Here's how the part is built. I have some questions about the finished solid (model axes, mm). A direction names the side the tool comes from. Give positions to 0.01 mm unless a question says otherwise; leave off trailing zeros. Order: outer loops, then holes, each group sorted by start corner. A loop starts at its lowest first (then second) coordinate and runs counter-clockwise, first axis right, second up.
from build123d import *

# Parameters (mm, degrees)
F0_W     = 180
F0_H     = 150
F1_DEPTH = 20
F2_R     = 4
F3_DEPTH = 10
F4_W     = 20
F4_H     = 150
F5_DEPTH = 10
F6_ANGLE = 90


with BuildPart() as f1:
    # F0 (on Front) → F1 (new body)
    with BuildSketch(Plane.XZ):
        with Locations((-90, 75)):
            Rectangle(F0_W, F0_H)
    extrude(amount=F1_DEPTH)

    # F2 (on face) → F3 (cut)
    with BuildSketch(Plane.XZ.offset(20)):
        with Locations((-10, 105)):
            Circle(F2_R)
        with Locations((-10, 75)):
            Circle(F2_R)
        with Locations((-10, 45)):
            Circle(F2_R)
    extrude(amount=-F3_DEPTH, mode=Mode.SUBTRACT)

    # F4 (on face) → F5 (cut)
    with BuildSketch(Plane.XZ.offset(20)):
        with Locations((-170, 75)):
            Rectangle(F4_W, F4_H)
    extrude(amount=-F5_DEPTH, mode=Mode.SUBTRACT)


with BuildPart() as f1_1:
    # F6: moved
    add(f1.part.rotate(Axis((-180, 0, 75), (0, 0, 1)), F6_ANGLE))


solid = f1_1.part
Q1. If we section it at A-A on x = -166: List the corners of the cut face in (y, z) for me.
Filled sheet:
outline: (20, 0) - (180, 0) - (180, 150) - (20, 150) - close; hole circle Ø8 at (170, 45); hole circle Ø8 at (170, 75); hole circle Ø8 at (170, 105)
Q2. Thinking about a two-plate mould opening in Y: for faces 4 (the face through (-164.93, 173.815, 46.201)), 5 (the face through (-170, 180, 74)), 6 (the face through (-165, 20, 74)), 7 (the face through (-160, 99, 76)), which applies, released by +Y, released by -Y, zero draft, split by the parting line, or undercut?
Filled sheet:
face 4: undercut
face 5: released by +Y
face 6: released by -Y
face 7: zero draft
Q3. If we section it at D-D on y = 13: List the corners of the cut face in (x, z) for me, plus the area to 3 significant figures.
Filled sheet:
outline: (-180, 0) - (-170, 0) - (-170, 150) - (-180, 150) - close
area: 1,500 mm2
Q4. If we section it at B-B on z = 75: List the corners of the cut face in (x, y) for me.
Filled sheet:
outline: (-180, 0) - (-170, 0) - (-170, 20) - (-160, 20) - (-160, 166) - (-170, 166) - (-170, 174) - (-160, 174) - (-160, 180) - (-180, 180) - close
Q5. For faces 1 (the face through (-170, 10, 76)), 2 (the face through (-170, 89, 0)), 3 (the face through (-170, 170, 45)), which set-ups out of +Z, -Z, +X, -X, +Y, -Y let a thin tool reach every point of the face, with its end or its side?
Filled sheet:
face 1: +Z, -Z, +X, -Y
face 2: -Z, +X, -X, +Y, -Y
face 3: +X
Q6. I need wall thicknesses on L1, parallel to Z at x = -167, y = 170; L2, parallel to Y at x = -165.25, z = 104.5; L3, parallel to Z at x = -169.5, y = 171.5. Which ranges of each line are inside material? Lowest first, please.
Filled sheet:
L1: z = 0 to 41, 49 to 71, 79 to 101, 109 to 150
L2: y = 20 to 166.03, 173.97 to 180
L3: z = 0 to 41.29, 48.71 to 71.29, 78.71 to 101.29, 108.71 to 150
Q7. I'm going to push flat-ended pins straight in: P1, Ø22, axis at y = 5.5, z = 66.5, coming from the +X side; P2, Ø3, axis at x = -165.5, z = 78.5, coming from the -Y side. Where does each tip first touch, or does it pass through?
Filled sheet:
P1: stops at x = -170
P2: stops at y = 20
Q8. If we section it at C-C on y = 170: List the corners of the cut face in (x, z) for me, plus the area to 3 significant figures.
Filled sheet:
outline: (-180, 0) - (-160, 0) - (-160, 41) - (-170, 41) - (-170, 49) - (-160, 49) - (-160, 71) - (-170, 71) - (-170, 79) - (-160, 79) - (-160, 101) - (-170, 101) - (-170, 109) - (-160, 109) - (-160, 150) - (-180, 150) - close
area: 2,760 mm2
